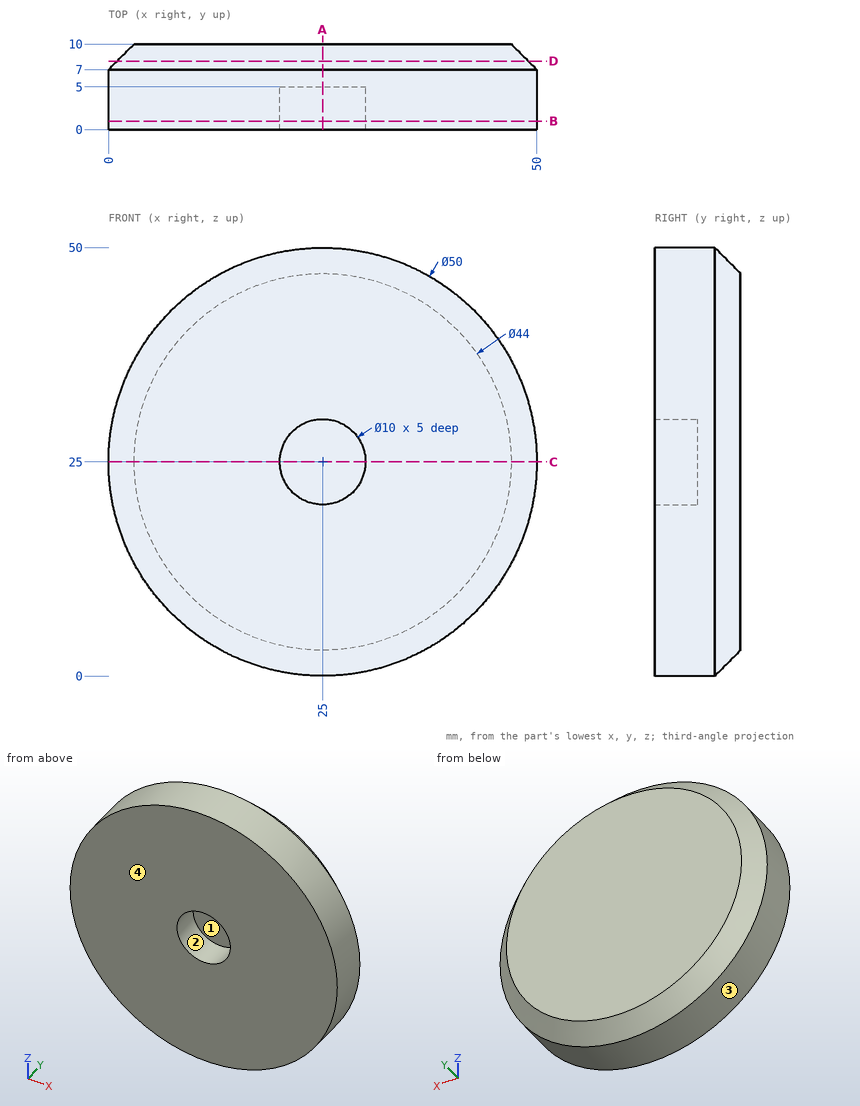
Geometry check sheet. Reference: drawing and pictorial views, mm from the part's lowest x, y, z. Coordinates: 2 decimals unless noted, no trailing zeros. Loops run counter-clockwise (first coordinate to the right, second up) from the corner with the lowest first, then second, coordinate; pieces in that order, holes last. Notation, with made-up numbers: (73.5, 14) -> (110.5, 14) arc R25 ccw to (110.5, 46) -> close; hole circle Ø2 at (17, 9). An arc over 180 degrees is marked (long way). Put each result on its own line as item: value.
1) Thickness scan on line 1 (Z direction, x = 25, y = 3.4); line 2 (Z direction, x = 14, y = 7); line 3 (Z direction, x = 4, y = 6). Record the ranges inside material, lowest first.
Result set:
line 1: z = 0 to 20, 30 to 50
line 2: z = 2.55 to 47.45
line 3: z = 11.44 to 38.56
2) Cross-section at A-A on x = 25. Record the boundary of the cut face in (y, z).
Result set:
outline: (0, 0) -> (7, 0) -> (10, 3) -> (10, 47) -> (7, 50) -> (0, 50) -> (0, 30) -> (5, 30) -> (5, 20) -> (0, 20) -> close
3) Gauge pin test, flat ends, axial feed: pin 1 Ø1.5 at (x, z) = (43, 40) entering from +Y; pin 2 Ø4 at (y, z) = (7, 15) entering from +X; pin 3 Ø6 at (x, z) = (25, 25) entering from -Y. Record the tip position at first contact, or that the pin passes through.
Result set:
pin 1: stops at y = 9.32
pin 2: stops at x = 48.69
pin 3: stops at y = 5
4) Cross-section at D-D on y = 8. Record the boundary of the cut face in (x, z), plus the area to 3 significant figures.
Result set:
outline: circle Ø48 at (25, 25)
area: 1,810 mm^2
5) Release check for a two-part mould opening along Z. For the marked faces 1, 2, 3 and 4 record: released by +Z, released by -Z, zero draft, split by the parting line, or undercut.
Result set:
face 1: undercut
face 2: undercut
face 3: split by the parting line
face 4: zero draft
6) Cross-section at B-B on y = 1. Record the boundary of the cut face in (x, z).
Result set:
outline: circle Ø50 at (25, 25); hole circle Ø10 at (25, 25)
7) Cross-section at C-C on z = 25. Record the boundary of the cut face in (x, y).
Result set:
outline: (0, 0) -> (20, 0) -> (20, 5) -> (30, 5) -> (30, 0) -> (50, 0) -> (50, 7) -> (47, 10) -> (3, 10) -> (0, 7) -> close
